from build123d import *

# Parameters (mm, degrees)
SKETCH1_W           = 28
SKETCH1_H           = 55
BOSS_EXTRUDE1_DEPTH = 40
SKETCH3_W           = 40
SKETCH3_H           = 60
BOSS_EXTRUDE2_DEPTH = 1
SKETCH4_W           = 40
SKETCH4_H           = 60
BOSS_EXTRUDE3_DEPTH = 1
SKETCH5_R           = 1.5
CUT_EXTRUDE1_DEPTH  = 53.46189093
SKETCH6_R           = 4
BOSS_EXTRUDE4_DEPTH = 4
SKETCH7_R           = 3.5
BOSS_EXTRUDE5_DEPTH = 1


with BuildPart() as part:
    # Sketch1 → Boss-Extrude1 (new body)
    with BuildSketch(Plane.XY):
        with Locations((-6e-08, 0)):
            Rectangle(SKETCH1_W, SKETCH1_H)
    extrude(amount=BOSS_EXTRUDE1_DEPTH)

    # Sketch3 → Boss-Extrude2 (add)
    with BuildSketch(Plane.XY.offset(36)):
        with Locations((0, -2.5)):
            Rectangle(SKETCH3_W, SKETCH3_H)
    extrude(amount=-BOSS_EXTRUDE2_DEPTH)

    # Sketch4 → Boss-Extrude3 (add)
    with BuildSketch(Plane(origin=(0, 0, 4), x_dir=(-1, 0, 0), z_dir=(0, 0, -1))):
        with Locations((0, -2.5)):
            Rectangle(SKETCH4_W, SKETCH4_H)
    extrude(amount=-BOSS_EXTRUDE3_DEPTH)

    # Sketch5 → Cut-Extrude1 (cut, through all)
    with BuildSketch(Plane.XY.offset(36)):
        with Locations(Location((-17, 19, 0), (0, 0, 180))):
            Circle(SKETCH5_R)
        with Locations(Location((17, 18.999999934, 0), (0, 0, 180))):
            Circle(SKETCH5_R)
        with Locations(Location((-17, -3, 0), (0, 0, 180))):
            Circle(SKETCH5_R)
        with Locations(Location((17, -3.000000066, 0), (0, 0, 180))):
            Circle(SKETCH5_R)
        with Locations(Location((17, -25.000000066, 0), (0, 0, 180))):
            Circle(SKETCH5_R)
        with Locations(Location((-17, -25, 0), (0, 0, 180))):
            Circle(SKETCH5_R)
    extrude(amount=-CUT_EXTRUDE1_DEPTH, mode=Mode.SUBTRACT)

    # Sketch6 → Boss-Extrude4 (add)
    with BuildSketch(Plane.XY.offset(40)):
        with Locations((0, 14.5)):
            Circle(SKETCH6_R)
    extrude(amount=BOSS_EXTRUDE4_DEPTH)

    # Sketch7 → Boss-Extrude5 (add)
    with BuildSketch(Plane(origin=(0, 0, 0), x_dir=(-1, 0, 0), z_dir=(0, 0, -1))):
        with Locations(Location((0, 13.5, 0), (0, 0, 180))):
            Circle(SKETCH7_R)
    extrude(amount=BOSS_EXTRUDE5_DEPTH)


solid = part.part
Here's how the part is built. I have some questions about the finished solid (model axes, mm). A direction names the side the tool comes from. Round coordinates to 2 decimals unless told otherwise and drop trailing zeros. Loops run counter-clockwise (first coordinate to the right, second up) from the corner with the lowest first, then second, coordinate; pieces in that order, holes last. Notation, with made-up numbers: (78, 17.25) - (137, 17.25) arc R13 cw to (137, 30.25) - close; hole circle Ø9 at (46.5, 58.5). An arc over 180 degrees is marked (long way). One line per question, with ' | ' between items. Start each with the question number.
Q1. Will these pins go through, and if not, where does the flat tip stop? pin 1 (5 mm diameter, centred on x = 17, y = -25, fed in from -Z); pin 2 (9 mm diameter, centred on y = 5.5, z = 24.5, fed in from +X); pin 3 (5 mm diameter, centred on x = -7.5, y = 9.5, fed in from -Z).
Q2. I want a section at C-C (x = -12). Write out the boundary of the cut face in (y, z).
Q3. I want a section at A-A (x = -17). State how many separate pieces and enclosed holes the cut face has, then the cut area to 3 significant figures.
Q4. I want a section at B-B (y = 1). Write out the boundary of the cut face in (x, z).
Q5. We'd pull the mould along Z, two halves only. Please class faces 5 (the flat face through (14, 0, 38)), 6 (the flat face through (0, 0, 40)), 7 (the flat face through (15, -5, 5)), 8 (the flat face through (0, 0, 0)): +Z half, -Z half, draft (parallel to the pull), parting line (faces both ways), or undercut.
Q6. I want a section at D-D (z = 13.5). Write out the boundary of the cut face in (x, y).
Q7. For faces 1 (the flat face through (-15, -5, 35)), 2 (the flat face through (0, -27.5, 38)), 3 (the flat face through (0, -27.5, 2)), 4 (the flat face through (14, 0, 20)), which set-ups out of +Z, -Z, +X, -X, +Y, -Y let a thin tool reach every point of the face, with its end or its side?
Q8. Please list where these lines run through material, in increasing order: line 1 (X direction, y = 19, z = 35.5); line 2 (Y direction, x = -17, z = 4.6); line 3 (Z direction, x = 14.5, y = 10.5). Write a range as [from, to].
Response values:
1) pin 1: stops at z = 4 | pin 2: stops at x = 14 | pin 3: stops at z = 0
2) outline: (-32.5, 4) - (-27.5, 4) - (-27.5, 0) - (27.5, 0) - (27.5, 40) - (-27.5, 40) - (-27.5, 36) - (-32.5, 36) - (-32.5, 35) - (-27.5, 35) - (-27.5, 5) - (-32.5, 5) - close
3) separate pieces: 8 | enclosed holes: 0 | area: 102 mm²
4) outline: (-20, 4) - (-14, 4) - (-14, 0) - (14, 0) - (14, 4) - (20, 4) - (20, 5) - (14, 5) - (14, 35) - (20, 35) - (20, 36) - (14, 36) - (14, 40) - (-14, 40) - (-14, 36) - (-20, 36) - (-20, 35) - (-14, 35) - (-14, 5) - (-20, 5) - close
5) face 5: draft | face 6: +Z half | face 7: undercut | face 8: -Z half
6) outline: (-14, -27.5) - (14, -27.5) - (14, 27.5) - (-14, 27.5) - close
7) face 1: -Y | face 2: +Z, +X, -X, -Y | face 3: -Z, +X, -X, -Y | face 4: +X, +Y, -Y
8) line 1: x = [-20, -18.5], [-15.5, 15.5], [18.5, 20] | line 2: y = [-32.5, -26.5], [-23.5, -4.5], [-1.5, 17.5], [20.5, 27.5] | line 3: z = [4, 5], [35, 36]
